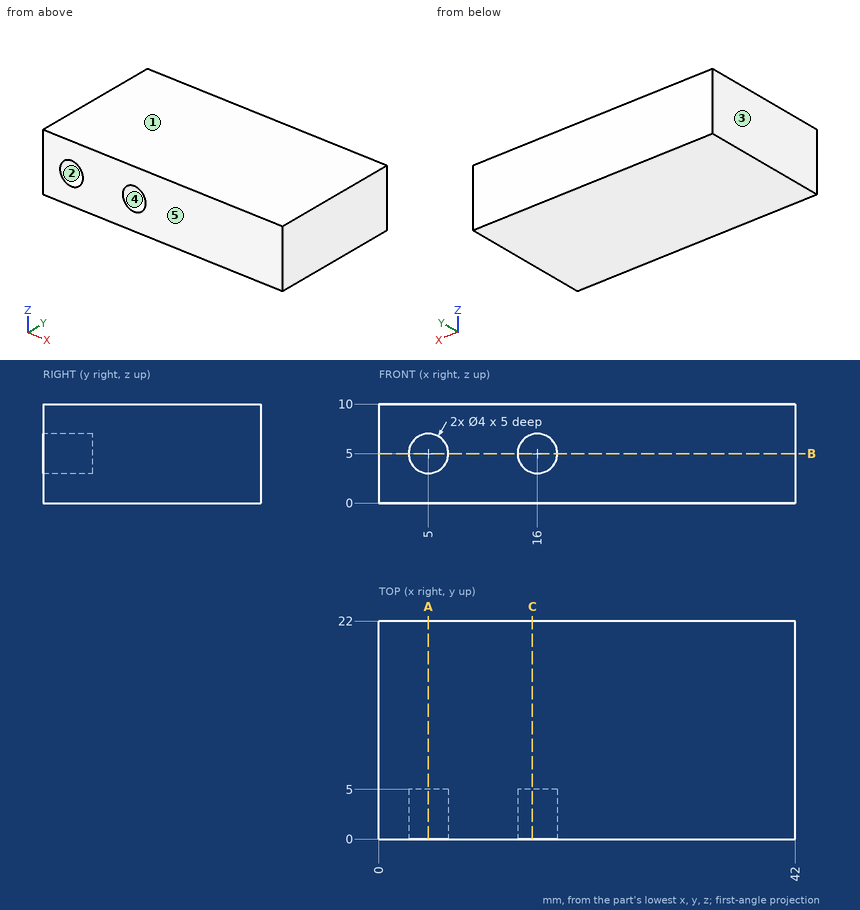
The drawing under review shows one solid part. Ordinate dimensions are in mm from its lowest x, y, z. A direction names the side the tool comes from. Round coordinates to 2 decimals unless told otherwise and drop trailing zeros. Write each loop counter-clockwise with the first axis right and the second up, starting at its lowest first coordinate (ties: lowest second). Pieces come first, ordered by that corner, then holes. Notation, with made-up numbers: M 15,64.25 L 44,64.25 A14 cw 44,82.25 Z; hole C -11,88.25 d5. An arc over 180 degrees is marked long. One line per item, written item: value. Start each with the question number.
(1) We need section A-A (x = 5). Give the boundary of the cut face in (y, z), and give its area (3 significant figures).
(2) The part is to be moulded in two halves that separate along X. For the marked faces 3, 4 and 5, say which applies: released by +X, released by -X, zero draft, split by the parting line, or undercut.
(3) We need section C-C (x = 15.5). Give the boundary of the cut face in (y, z), and give its area (3 significant figures).
(4) Wall thickness on line 1 (X direction, y = 2.4, z = 5): over which ranges is the line inside the solid? List them lowest first.
(5) We need section B-B (z = 5). Give the boundary of the cut face in (x, y).
(6) Machinability: for the marked faces 1 and 2, which of the approach directions +Z, -Z, +X, -X, +Y, -Y give a long, thin tool a straight path to every point of the face, cutting with its end or side? Answer none if there is none.
Result:
1. outline: M 0,0 L 22,0 L 22,10 L 0,10 L 0,7 L 5,7 L 5,3 L 0,3 Z
1. area: 200 mm²
2. face 3: released by -X
2. face 4: undercut
2. face 5: zero draft
3. outline: M 0,0 L 22,0 L 22,10 L 0,10 L 0,6.94 L 5,6.94 L 5,3.06 L 0,3.06 Z
3. area: 201 mm²
4. line 1: 0 to 3, 7 to 14, 18 to 42
5. outline: M 0,0 L 3,0 L 3,5 L 7,5 L 7,0 L 14,0 L 14,5 L 18,5 L 18,0 L 42,0 L 42,22 L 0,22 Z
6. face 1: +Z, +X, -X, +Y, -Y
6. face 2: -Y
